```python
from build123d import *

# Parameters (mm, degrees)
BOSS_EXTRUDE1_DEPTH = 3.175
SKETCH2_W           = 3.175
SKETCH2_H           = 8.466666667
CUT_EXTRUDE1_DEPTH  = 3.175
SKETCH3_W           = 3.175
SKETCH3_H           = 12.7
BOSS_EXTRUDE2_DEPTH = 3.175
CUT_EXTRUDE2_DEPTH  = 3.175
SKETCH5_W           = 12.7
SKETCH5_H           = 3.175
CUT_EXTRUDE3_DEPTH  = 3.175
SKETCH6_W           = 12.7
SKETCH6_H           = 3.175
CUT_EXTRUDE4_DEPTH  = 3.175
CUT_EXTRUDE5_DEPTH  = 3.175


with BuildPart() as part:
    # Sketch1 → Boss-Extrude1 (new body)
    with BuildSketch(Plane(origin=(0, 0, 0), x_dir=(0, 0, -1), z_dir=(1, 0, 0))):
        with BuildLine():
            Line((-201.6125, -203.2), (201.6125, -203.2))
            Line((201.6125, -203.2), (201.6125, 127))
            ThreePointArc((201.6125, 127), (179.294036726, 180.881536726), (125.4125, 203.2))
            Line((125.4125, 203.2), (-125.4125, 203.2))
            ThreePointArc((-125.4125, 203.2), (-179.294036726, 180.881536726), (-201.6125, 127))
            Line((-201.6125, 127), (-201.6125, -203.2))
        make_face()
    extrude(amount=BOSS_EXTRUDE1_DEPTH)

    # Sketch2 → Cut-Extrude1 (cut)
    with BuildSketch(Plane(origin=(3.175, 0, 0), x_dir=(0, 0, -1), z_dir=(1, 0, 0))):
        with Locations((-3.175, 110.066666667)):
            Rectangle(SKETCH2_W, SKETCH2_H)
        with Locations((196.85, 110.066666667)):
            Rectangle(SKETCH2_W, SKETCH2_H)
        with Locations((196.85, 93.133333334)):
            Rectangle(SKETCH2_W, SKETCH2_H)
        with Locations((-3.175, 93.133333334)):
            Rectangle(SKETCH2_W, SKETCH2_H)
    extrude(amount=-CUT_EXTRUDE1_DEPTH, mode=Mode.SUBTRACT)

    # Sketch3 → Boss-Extrude2 (add)
    with BuildSketch(Plane.XY.offset(201.6125)):
        with Locations((1.5875, 101.6)):
            Rectangle(SKETCH3_W, SKETCH3_H)
    extrude(amount=BOSS_EXTRUDE2_DEPTH)

    # Sketch4 → Cut-Extrude2 (cut)
    with BuildSketch(Plane(origin=(3.175, 0, 0), x_dir=(0, 0, -1), z_dir=(1, 0, 0))):
        with BuildLine():
            Line((-168.275, 76.941959208), (-168.275, -12.7))
            ThreePointArc((-168.275, -12.7), (-160.835512242, -30.660512242), (-142.875, -38.1))
            Line((-142.875, -38.1), (-66.675, -38.1))
            ThreePointArc((-66.675, -38.1), (-48.714487758, -30.660512242), (-41.275, -12.7))
            Line((-41.275, -12.7), (-41.275, 76.941959208))
            ThreePointArc((-41.275, 76.941959208), (-44.160306385, 88.699874475), (-52.160714286, 97.786515097))
            ThreePointArc((-52.160714286, 97.786515097), (-104.775, 114.3), (-157.389285714, 97.786515097))
            ThreePointArc((-157.389285714, 97.786515097), (-165.389693615, 88.699874475), (-168.275, 76.941959208))
        make_face()
        with BuildLine():
            Line((168.275, 76.941959208), (168.275, -12.7))
            ThreePointArc((168.275, -12.7), (160.835512242, -30.660512242), (142.875, -38.1))
            Line((142.875, -38.1), (66.675, -38.1))
            ThreePointArc((66.675, -38.1), (48.714487758, -30.660512242), (41.275, -12.7))
            Line((41.275, -12.7), (41.275, 76.941959208))
            ThreePointArc((41.275, 76.941959208), (44.160306385, 88.699874475), (52.160714286, 97.786515097))
            ThreePointArc((52.160714286, 97.786515097), (104.775, 114.3), (157.389285714, 97.786515097))
            ThreePointArc((157.389285714, 97.786515097), (165.389693615, 88.699874475), (168.275, 76.941959208))
        make_face()
    extrude(amount=-CUT_EXTRUDE2_DEPTH, mode=Mode.SUBTRACT)

    # Sketch5 → Cut-Extrude3 (cut)
    with BuildSketch(Plane(origin=(3.175, 0, 0), x_dir=(0, 0, -1), z_dir=(1, 0, 0))):
        with Locations((-188.9125, -195.2625)):
            Rectangle(SKETCH5_W, SKETCH5_H)
        with Locations((-163.5125, -195.2625)):
            Rectangle(SKETCH5_W, SKETCH5_H)
        with Locations((-138.1125, -195.2625)):
            Rectangle(SKETCH5_W, SKETCH5_H)
    cut_extrude3 = extrude(amount=-CUT_EXTRUDE3_DEPTH, mode=Mode.SUBTRACT)

    # Mirror1: Cut-Extrude3 across plane
    add(cut_extrude3.mirror(Plane.XY), mode=Mode.SUBTRACT)

    # Sketch6 → Cut-Extrude4 (cut)
    with BuildSketch(Plane(origin=(3.175, 0, 0), x_dir=(0, 0, -1), z_dir=(1, 0, 0))):
        with Locations((-25.4, -195.2625)):
            Rectangle(SKETCH6_W, SKETCH6_H)
        with Locations((0, -195.2625)):
            Rectangle(SKETCH6_W, SKETCH6_H)
        with Locations((25.4, -195.2625)):
            Rectangle(SKETCH6_W, SKETCH6_H)
    extrude(amount=-CUT_EXTRUDE4_DEPTH, mode=Mode.SUBTRACT)

    # Sketch7 → Cut-Extrude5 (cut)
    with BuildSketch(Plane(origin=(3.175, 0, 0), x_dir=(0, 0, -1), z_dir=(1, 0, 0))):
        with BuildLine():
            ThreePointArc((-158.8125, 152.4), (-158.926680701, 152.974025149), (-159.251839828, 153.460660172))
            Line((-159.251839828, 153.460660172), (-160.3125, 152.4))
            Line((-160.3125, 152.4), (-159.251839828, 151.339339828))
            ThreePointArc((-159.251839828, 151.339339828), (-158.926680701, 151.825974851), (-158.8125, 152.4))
        make_face()
        with BuildLine():
            Line((-160.3125, 152.4), (-159.251839828, 153.460660172))
            ThreePointArc((-159.251839828, 153.460660172), (-161.8125, 152.4), (-159.251839828, 151.339339828))
            Line((-159.251839828, 151.339339828), (-160.3125, 152.4))
        make_face()
        with BuildLine():
            Line((-149.751839828, 160.839339828), (-150.8125, 161.9))
            Line((-150.8125, 161.9), (-151.873160172, 160.839339828))
            ThreePointArc((-151.873160172, 160.839339828), (-150.8125, 160.4), (-149.751839828, 160.839339828))
        make_face()
        with BuildLine():
            Line((-151.873160172, 160.839339828), (-150.8125, 161.9))
            Line((-150.8125, 161.9), (-149.751839828, 160.839339828))
            ThreePointArc((-149.751839828, 160.839339828), (-149.426680701, 161.325974851), (-149.3125, 161.9))
            ThreePointArc((-149.3125, 161.9), (-151.386525149, 163.285819299), (-151.873160172, 160.839339828))
        make_face()
        with BuildLine():
            ThreePointArc((-139.8125, 152.4), (-140.738474851, 153.785819299), (-142.373160172, 153.460660172))
            Line((-142.373160172, 153.460660172), (-141.3125, 152.4))
            Line((-141.3125, 152.4), (-142.373160172, 151.339339828))
            ThreePointArc((-142.373160172, 151.339339828), (-140.738474851, 151.014180701), (-139.8125, 152.4))
        make_face()
        with BuildLine():
            Line((-141.3125, 152.4), (-142.373160172, 153.460660172))
            ThreePointArc((-142.373160172, 153.460660172), (-142.8125, 152.4), (-142.373160172, 151.339339828))
            Line((-142.373160172, 151.339339828), (-141.3125, 152.4))
        make_face()
        with BuildLine():
            ThreePointArc((-149.751839828, 143.960660172), (-150.8125, 144.4), (-151.873160172, 143.960660172))
            Line((-151.873160172, 143.960660172), (-150.8125, 142.9))
            Line((-150.8125, 142.9), (-149.751839828, 143.960660172))
        make_face()
        with BuildLine():
            Line((-150.8125, 142.9), (-151.873160172, 143.960660172))
            ThreePointArc((-151.873160172, 143.960660172), (-151.386525149, 141.514180701), (-149.3125, 142.9))
            ThreePointArc((-149.3125, 142.9), (-149.426680701, 143.474025149), (-149.751839828, 143.960660172))
            Line((-149.751839828, 143.960660172), (-150.8125, 142.9))
        make_face()
    cut_extrude5 = extrude(amount=-CUT_EXTRUDE5_DEPTH, mode=Mode.SUBTRACT)

    # Mirror2: Cut-Extrude5 across plane
    add(cut_extrude5.mirror(Plane.XY), mode=Mode.SUBTRACT)


solid = part.part
```
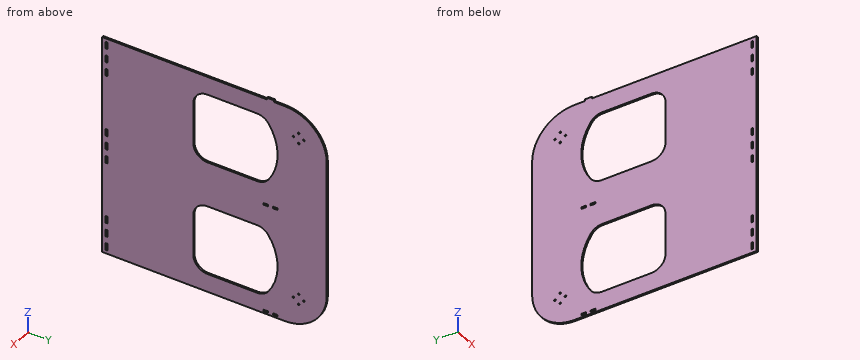
Part model, mm, in its own coordinate system. Round coordinates to 2 decimals unless told otherwise and drop trailing zeros. Write each loop counter-clockwise with the first axis right and the second up, starting at its lowest first coordinate (ties: lowest second). Pieces come first, ordered by that corner, then holes. Notation, with made-up numbers: (68.25, -13) -> (85.25, -13) arc R15 cw to (85.25, 13) -> close; hole circle Ø6 at (-9.5, -11). An arc over 180 degrees is marked (long way). Return JSON: item names as keys, results as strings. Group by question number.
Q1. Saw through at A-A on y = 56.5. Write the cut outline in (x, z) (1 decimal), plus the area to 3 significant figures.
Q2. Probe L1, parallel to Z at x = 0.5, y = -5 (1 decimal); L2, parallel to Y at x = 2.05, z = 0 (3 decimals); L3, parallel to Z at x = 2.4, y = 100. List the from-to ranges inside material, lowest first. Write a range as [from, to].
Q3. Saw through at C-C on x = 0.5. State how many separate pieces and enclosed holes the cut face has, plus the area to 3 significant figures.
Q4. Pin check, flat tips, straight feed: pin 1 (1.6 mm diameter, centred on x = 2, z = -185.5, fed in from +Y); pin 2 (1.6 mm diameter, centred on x = 2, y = -195, fed in from +Z); pin 3 (8 mm diameter, centred on y = 58, z = -44, fed in from -X); pin 4 (1.6 mm diameter, centred on x = 2, z = 161.5, fed in from +Y). Stop position of each tip, or through.
Q5. Saw through at D-D on z = 75. Write the cut outline in (x, y) (3 decimals).
Q6. Saw through at B-B on z = -78.5. Write the cut outline in (x, y) (3 decimals), plus the area to 3 significant figures.
Answer:
{
 "1": {"outline": "(0, -201.6) -> (3.2, -201.6) -> (3.2, -168.3) -> (0, -168.3) -> close; (0, -41.3) -> (3.2, -41.3) -> (3.2, 41.3) -> (0, 41.3) -> close; (0, 168.3) -> (3.2, 168.3) -> (3.2, 201.6) -> (0, 201.6) -> close", "area": "474 mm2"},
 "2": {"L1": "[-201.6, -168.3], [-41.3, 41.3], [168.3, 201.6]", "L2": "[-203.2, -196.85], [-193.675, 203.2]", "L3": "[-201.61, -154.06], [-55.49, 55.49], [154.06, 204.79]"},
 "3": {"separate pieces": "1", "enclosed holes": "23", "area": "125,000 mm2"},
 "4": {"pin 1": "y = 174.87", "pin 2": "z = 201.61", "pin 3": "x = 0", "pin 4": "y = 194.54"},
 "5": {"outline": "(0, -203.2) -> (3.175, -203.2) -> (3.175, -38.1) -> (0, -38.1) -> close; (0, 109.353) -> (3.175, 109.353) -> (3.175, 203.2) -> (0, 203.2) -> close"},
 "6": {"outline": "(0, -203.2) -> (3.175, -203.2) -> (3.175, -38.1) -> (0, -38.1) -> close; (0, 110.471) -> (3.175, 110.471) -> (3.175, 203.2) -> (0, 203.2) -> close", "area": "819 mm2"}
}
